Can you work these out from the drawing? Everything is in mm from the part's minimum corner. A direction names the side the tool comes from. Coordinates: 2 decimals unless noted, no trailing zeros. Order: outer loops, then holes, each group sorted by start corner. A loop starts at its lowest first (then second) coordinate and runs counter-clockwise, first axis right, second up. Notation, with made-up numbers: (23, 61.5) -> (39, 61.5) arc R17 cw to (39, 93.5) -> close; hole circle Ø8 at (79.5, -16). An arc over 180 degrees is marked (long way). Put each result on its own line as item: value. Start each with the question number.
Q1. Will these pins go through, and if not, where does the flat tip stop? pin 1 (1.8 mm diameter, centred on x = 8, y = 13.5, fed in from -Z); pin 2 (1.4 mm diameter, centred on y = 8.5, z = 3, fed in from +X); pin 3 (0.5 mm diameter, centred on x = 7.5, z = 2, fed in from -Y); pin 4 (1.4 mm diameter, centred on y = 6.5, z = 2, fed in from -X).
Q2. If we section it at D-D (y = 13.5): Please give me the cut outline in (x, z).
Q3. Please list where these lines run through material, in increasing order: line 1 along Y through (x, z) = (8, 0.75); line 2 along Z through (x, y) = (12, 12.75); line 3 along X through (y, z) = (6.75, 2.15).
Q4. If we section it at A-A (x = 8): Please give me the cut outline in (y, z).
Q5. If we section it at B-B (y = 9.25): Please give me the cut outline in (x, z).
Q6. For the marked faces 5 and 6, which set-ups out of +Z, -Z, +X, -X, +Y, -Y let a thin tool reach every point of the face, with its end or its side?
Q7. If we section it at C-C (z = 0.5): Please give me the cut outline in (x, y) (1 decimal).
Q8. We'd pull the mould along X, two halves only. Please class the marked faces 1, 2, 3 and 4: +X half, -X half, draft (parallel to the pull), parting line (faces both ways), or undercut.
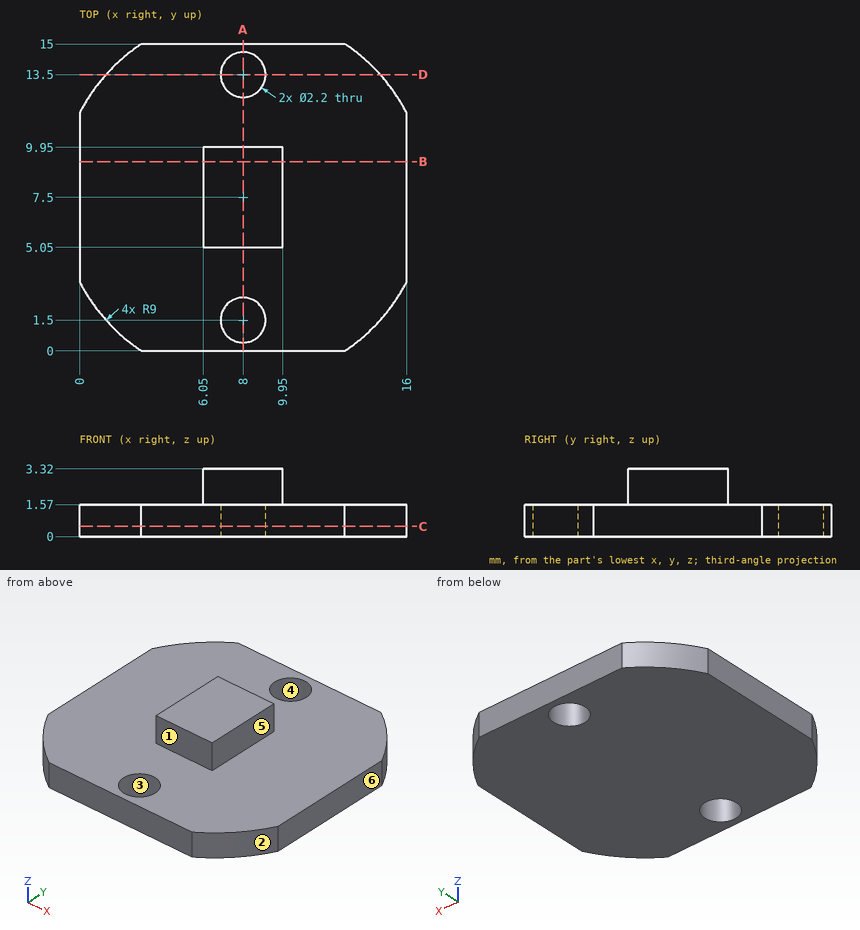
The answers:
1. pin 1: through
1. pin 2: x = 9.95
1. pin 3: y = 5.05
1. pin 4: x = 0
2. outline: (1.29, 0) -> (6.9, 0) -> (6.9, 1.57) -> (1.29, 1.57) -> close; (9.1, 0) -> (14.71, 0) -> (14.71, 1.57) -> (9.1, 1.57) -> close
3. line 1: 0 to 0.4, 2.6 to 12.4, 14.6 to 15
3. line 2: 0 to 1.57
3. line 3: 6.05 to 9.95
4. outline: (0, 0) -> (0.4, 0) -> (0.4, 1.57) -> (0, 1.57) -> close; (2.6, 0) -> (12.4, 0) -> (12.4, 1.57) -> (9.95, 1.57) -> (9.95, 3.32) -> (5.05, 3.32) -> (5.05, 1.57) -> (2.6, 1.57) -> close; (14.6, 0) -> (15, 0) -> (15, 1.57) -> (14.6, 1.57) -> close
5. outline: (0, 0) -> (16, 0) -> (16, 1.57) -> (9.95, 1.57) -> (9.95, 3.32) -> (6.05, 3.32) -> (6.05, 1.57) -> (0, 1.57) -> close
6. face 5: +Z, +X, +Y, -Y
6. face 6: +Z, -Z, +X, +Y, -Y
7. outline: (0, 3.4) arc R9 ccw to (3, 0) -> (13, 0) arc R9 ccw to (16, 3.4) -> (16, 11.6) arc R9 ccw to (13, 15) -> (3, 15) arc R9 ccw to (0, 11.6) -> close; hole circle Ø2.2 at (8, 1.5); hole circle Ø2.2 at (8, 13.5)
8. face 1: draft
8. face 2: +X half
8. face 3: undercut
8. face 4: undercut
